```python
from build123d import *

# Parameters (mm, degrees)
SKETCH1_W           = 95.25
SKETCH1_H           = 95.25
BOSS_EXTRUDE1_DEPTH = 38.1
SHELL1_T            = -6.35
BOSS_EXTRUDE2_DEPTH = 31.75
SKETCH3_R           = 1.905
SKETCH3_R_2         = 1.016
BOSS_EXTRUDE3_DEPTH = 6.35
SKETCH4_R           = 1.016
BOSS_EXTRUDE4_DEPTH = 8.89
SKETCH5_R           = 1.905
SKETCH5_W           = 31.75
SKETCH5_H           = 5.08
BOSS_EXTRUDE5_DEPTH = 6.35
SKETCH7_R           = 1.016
BOSS_EXTRUDE6_DEPTH = 8.89
SKETCH8_R           = 2.38125
CUT_EXTRUDE1_DEPTH  = 8.89
BOSS_EXTRUDE7_DEPTH = 6.35


with BuildPart() as part:
    # Sketch1 → Boss-Extrude1 (new body)
    with BuildSketch(Plane.XY):
        Rectangle(SKETCH1_W, SKETCH1_H)
    extrude(amount=BOSS_EXTRUDE1_DEPTH)

    # Shell1
    shell1_openings = [part.faces().sort_by_distance(p)[0] for p in [
        (0, 0, 38.1),
    ]]
    offset(amount=SHELL1_T, openings=shell1_openings, kind=Kind.INTERSECTION)

    # Sketch2 → Boss-Extrude2 (add)
    with BuildSketch(Plane.XY.offset(38.1)):
        with BuildLine():
            Line((-41.275, 41.275), (-36.195, 41.275))
            ThreePointArc((-36.195, 41.275), (-37.682897552, 37.682897552), (-41.275, 36.195))
            Line((-41.275, 36.195), (-41.275, 41.275))
        make_face()
        with BuildLine():
            Line((36.195, 41.275), (41.275, 41.275))
            Line((41.275, 41.275), (41.275, 36.195))
            ThreePointArc((41.275, 36.195), (37.682897552, 37.682897552), (36.195, 41.275))
        make_face()
        with BuildLine():
            Line((41.275, -36.195), (41.275, -41.275))
            Line((41.275, -41.275), (36.195, -41.275))
            ThreePointArc((36.195, -41.275), (37.682897552, -37.682897552), (41.275, -36.195))
        make_face()
        with BuildLine():
            Line((-41.275, -36.195), (-41.275, -41.275))
            Line((-41.275, -41.275), (-36.195, -41.275))
            ThreePointArc((-36.195, -41.275), (-37.682897552, -37.682897552), (-41.275, -36.195))
        make_face()
    extrude(amount=-BOSS_EXTRUDE2_DEPTH)

    # Sketch3 → Boss-Extrude3 (add)
    with BuildSketch(Plane.XY.offset(6.35)):
        with Locations((35.015710728, 31.115)):
            Circle(SKETCH3_R)
        with Locations((-10.704289272, 31.115)):
            Circle(SKETCH3_R_2)
        with Locations((-10.704289272, 13.335)):
            Circle(SKETCH3_R)
        with Locations((35.015710728, 13.335)):
            Circle(SKETCH3_R)
    extrude(amount=BOSS_EXTRUDE3_DEPTH)

    # Sketch4 → Boss-Extrude4 (add)
    with BuildSketch(Plane.XY.offset(12.7)):
        with Locations((-10.704289272, 31.115)):
            Circle(SKETCH4_R)
        with Locations((-10.704289272, 13.335)):
            Circle(SKETCH4_R)
        with Locations((35.015710728, 31.115)):
            Circle(SKETCH4_R)
        with Locations((35.015710728, 13.335)):
            Circle(SKETCH4_R)
    extrude(amount=BOSS_EXTRUDE4_DEPTH)

    # Sketch5 → Boss-Extrude5 (add)
    with BuildSketch(Plane.XY.offset(6.35)):
        with Locations((5.715, -32.385)):
            Circle(SKETCH5_R)
        with Locations((33.655, -32.385)):
            Circle(SKETCH5_R)
        with Locations((19.685, 3.175)):
            Rectangle(SKETCH5_W, SKETCH5_H)
    extrude(amount=BOSS_EXTRUDE5_DEPTH)

    # Sketch7 → Boss-Extrude6 (add)
    with BuildSketch(Plane.XY.offset(12.7)):
        with Locations((5.715, -32.385)):
            Circle(SKETCH7_R)
        with Locations((33.655, -32.385)):
            Circle(SKETCH7_R)
    extrude(amount=BOSS_EXTRUDE6_DEPTH)

    # Sketch8 → Cut-Extrude1 (cut)
    with BuildSketch(Plane.XY.offset(38.1)):
        with Locations((-41.275, 41.275)):
            Circle(SKETCH8_R)
        with Locations((41.275, 41.275)):
            Circle(SKETCH8_R)
        with Locations((41.275, -41.275)):
            Circle(SKETCH8_R)
        with Locations((-41.275, -41.275)):
            Circle(SKETCH8_R)
    extrude(amount=-CUT_EXTRUDE1_DEPTH, mode=Mode.SUBTRACT)

    # Sketch10 → Boss-Extrude7 (add)
    with BuildSketch(Plane.XY.offset(6.35)):
        Polygon((-37.696932409, -30.607), (-37.696932409, 2.9972), (-1.781332409, 2.9972), (-1.781332409, -30.607), (-6.861332409, -30.607), (-6.861332409, -2.0828), (-32.616932409, -2.0828), (-32.616932409, -30.607), align=None)
    extrude(amount=BOSS_EXTRUDE7_DEPTH)


solid = part.part
```
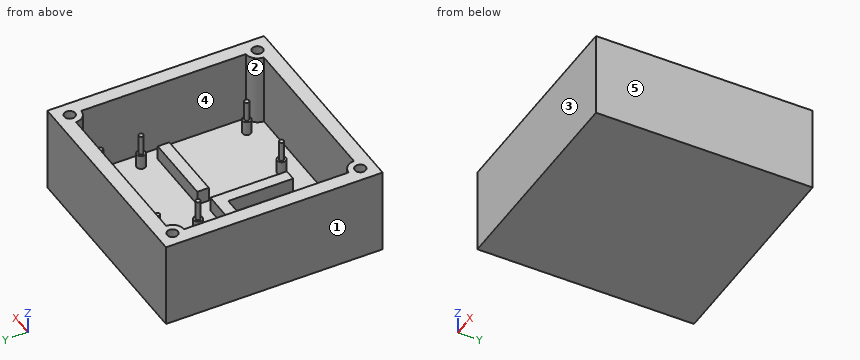
Input: part model. Units: mm. Frame: model coordinates. Face numbers are marked on the shaded views. A direction names the side the tool comes from. Give positions to 0.01 mm unless a question says otherwise; leave off trailing zeros. Write each loop counter-clockwise with the first axis right and the second up, starting at its lowest first coordinate (ties: lowest second). Pieces come first, ordered by that corner, then holes. Notation, with made-up numbers: (-10.75, 68.5) - (42.25, 68.5) arc R8 ccw to (42.25, 78.5) - close; hole circle Ø11 at (-9.75, -20). An arc over 180 degrees is marked (long way). Write item = value, one per line. Start each with the question number.
1. Section query D-D, the plane z = 8. Count the separate pieces of the cut face and the enclosed holes in it, then the cut area to 3 significant figures.
2. Mould query, pull axis X, two halves, no side actions, for the marked faces 1, 2 and 3. Classes: released by +X, released by -X, zero draft, split by the parting line, or undercut.
3. Ray query, L1, parallel to X at y = -19, z = 12.5 (3 decimals); L2, parallel to Y at x = -20.5, z = 10 (3 decimals); L3, parallel to X at y = -28, z = 35 (3 decimals). Return the intervals inside material, ascending.
4. Access query for the marked faces 4 and 5. Directions: +Z, -Z, +X, -X, +Y, -Y. A direction counts if a zero-diameter tool reaches every point of the face in a straight line with its end or side. Return the directions, or none.
5. Section query C-C, the plane z = 26. Output: boundary loops of the cut face in (x, y) (3 decimals).
6. Section query B-B, the plane y = 21. Output: boundary loops of the cut face in (x, z) (3 decimals).
7. First-contact query: pin 1 Ø1 at (x, y) = (-10.5, 13) entering from +Z; pin 2 Ø3 at (x, y) = (-41.275, -41.275) entering from +Z. Flat tips, straight axial feed; report the tip coordinate or a pass-through.
8. Section query A-A, the plane z = 16.5. Output: boundary loops of the cut face in (x, y) (3 decimals).
Check sheet entries:
q1.separate_pieces = 9
q1.enclosed_holes = 1
q1.area = 3,030 mm2
q2.face_1 = released by -X
q2.face_2 = undercut
q2.face_3 = zero draft
q3.L1 = -47.625 to -41.275, -37.697 to -32.617, -6.861 to -1.781, 41.275 to 47.625
q3.L2 = -47.625 to -41.275, -2.083 to 2.997, 41.275 to 47.625
q3.L3 = -47.625 to -41.275, 41.275 to 47.625
q4.face_4 = +Z
q4.face_5 = +Z, -Z, +X, +Y, -Y
q5.outline = (-47.625, -47.625) - (47.625, -47.625) - (47.625, 47.625) - (-47.625, 47.625) - close; hole (-41.275, -36.195) arc R5.08 cw to (-36.195, -41.275) - (36.195, -41.275) arc R5.08 cw to (41.275, -36.195) - (41.275, 36.195) arc R5.08 cw to (36.195, 41.275) - (-36.195, 41.275) arc R5.08 cw to (-41.275, 36.195) - close
q6.outline = (-47.625, 0) - (47.625, 0) - (47.625, 38.1) - (41.275, 38.1) - (41.275, 6.35) - (-41.275, 6.35) - (-41.275, 38.1) - (-47.625, 38.1) - close
q7.pin_1 = 21.59
q7.pin_2 = 29.21
q8.outline = (-47.625, -47.625) - (47.625, -47.625) - (47.625, 47.625) - (-47.625, 47.625) - close; circle Ø2.032 at (-10.704, 13.335); circle Ø2.032 at (-10.704, 31.115); circle Ø2.032 at (5.715, -32.385); circle Ø2.032 at (33.655, -32.385); circle Ø2.032 at (35.016, 13.335); circle Ø2.032 at (35.016, 31.115); hole (-41.275, -36.195) arc R5.08 cw to (-36.195, -41.275) - (36.195, -41.275) arc R5.08 cw to (41.275, -36.195) - (41.275, 36.195) arc R5.08 cw to (36.195, 41.275) - (-36.195, 41.275) arc R5.08 cw to (-41.275, 36.195) - close
